Model file for the job. Use its own axes, mm. A direction names the side the tool comes from. Coordinates: 2 decimals unless noted, no trailing zeros. Order: outer loops, then holes, each group sorted by start corner. A loop starts at its lowest first (then second) coordinate and runs counter-clockwise, first axis right, second up. Notation, with made-up numbers: (89, 52) -> (138, 52) arc R26 ccw to (138, 67) -> close; hole circle Ø1 at (88.5, -36). An arc over 180 degrees is marked (long way). Write item = value, one per line. Start each with the question number.
Q1. Cut at C-C, the plane y = 0.9. List the corners of the cut face in (x, z), plus the area to 3 significant figures.
Q2. 3-axis set-ups, long thin cutter, end or side, ignore diameter. For faces 1 (the face through (9.53, -0.85, 3.16)), 2 (the face through (0, -0.65, 4)): which of +Z, -Z, +X, -X, +Y, -Y reach the whole face in a straight line?
Q3. Cut at B-B, the plane x = 1. List the corners of the cut face in (y, z).
Q4. Cut at D-D, the plane z = 2.25. List the corners of the cut face in (x, y), plus the area to 3 significant figures.
Q5. Flat gauge pins, fed straight in: pin 1 (1 mm diameter, centred on y = 0.5, z = 7, fed in from -X); pin 2 (0.5 mm diameter, centred on x = 5, y = 0.5, fed in from +Z). Where does each tip first touch, or does it go through?
Q6. Cut at A-A, the plane z = 5.75. List the corners of the cut face in (x, y).
Q7. Wall check: line 1 (Y direction, x = -7.75, z = 3.5); line 2 (Z direction, x = 7.5, y = 0.45); line 3 (X direction, y = -0.25, z = -0.5). Give the ranges that are in metal, low to high. Write a range as from..to.
from build123d import *

# Parameters (mm, degrees)
PAD_DEPTH      = 12
PAD_DEPTH_BACK = 12
POCKET_DEPTH   = 2.501
FILLET_R       = 3
FILLET001_R    = 0.2


with BuildPart() as part:
    # Sketch → Pad (new body, two sides)
    with BuildSketch(Plane.YZ) as pad_sk:
        Polygon((0, 0), (0.65, 0), (0.65, 8.6), (1.25, 8.6), (1.25, -1), (0, -1), (-1.25, -1), (-1.25, 8.6), (-0.65, 8.6), (-0.65, -4e-06), align=None)
    extrude(amount=PAD_DEPTH)
    extrude(pad_sk.sketch, amount=-PAD_DEPTH_BACK)

    # Sketch001 (on Face7 of Pad) → Pocket (cut, through all)
    with BuildSketch(Plane(origin=(0, -1.25, 0), x_dir=(0, 0, -1), z_dir=(0, -1, 0))):
        Polygon((1, 12), (-8.6, 6.3), (-8.6, 0), (-8.6, -6.3), (1, -12), (1, -14), (-11, -14), (-11, 0), (-11, 14), (1, 14), align=None)
    extrude(amount=-POCKET_DEPTH, mode=Mode.SUBTRACT)

    # Fillet
    fillet_edges = [part.edges().sort_by_distance(p)[0] for p in [
        (6.3, -0.95, 8.6),
        (6.3, 0.95, 8.6),
        (-6.3, 0.95, 8.6),
        (-6.3, -0.95, 8.6),
    ]]
    fillet(fillet_edges, radius=FILLET_R)

    # Fillet001
    fillet001_edges = [part.edges().sort_by_distance(p)[0] for p in [
        (12, -0.625, -1),
        (12, 0.625, -1),
        (-12, 0.625, -1),
        (-12, -0.625, -1),
    ]]
    fillet(fillet001_edges, radius=FILLET001_R)


solid = part.part
Here are the results:
q1.outline = (-11.82, -0.7) arc R0.2 ccw to (-11.65, -1) -> (11.65, -1) arc R0.2 ccw to (11.82, -0.7) -> (7.17, 7.13) arc R3 ccw to (4.59, 8.6) -> (-4.59, 8.6) arc R3 ccw to (-7.17, 7.13) -> close
q1.area = 175 mm²
q2.face_1 = +Z, +X, +Y, -Y
q2.face_2 = +Z, +X, -X
q3.outline = (-1.25, -1) -> (1.25, -1) -> (1.25, 8.6) -> (0.65, 8.6) -> (0.65, 0) -> (0, 0) -> (-0.65, 0) -> (-0.65, 8.6) -> (-1.25, 8.6) -> close
q4.outline = (-10.07, -1.25) -> (10.07, -1.25) -> (10.07, -0.65) -> (-10.07, -0.65) -> close; (-10.07, 0.65) -> (10.07, 0.65) -> (10.07, 1.25) -> (-10.07, 1.25) -> close
q4.area = 24.2 mm²
q5.pin_1 = -7.53
q5.pin_2 = 8.59
q6.outline = (-7.99, -1.25) -> (7.99, -1.25) -> (7.99, -0.65) -> (-7.99, -0.65) -> close; (-7.99, 0.65) -> (7.99, 0.65) -> (7.99, 1.25) -> (-7.99, 1.25) -> close
q7.line_1 = -1.25..-0.65, 0.65..1.25
q7.line_2 = -1..0
q7.line_3 = -11.7..11.7
